Source: CAD feature listing. Evaluate the final solid. Frame: model axes, mm. Face numbers are marked on the shaded views. A direction names the side the tool comes from. Round coordinates to 2 decimals unless told otherwise and drop trailing zeros. Loops run counter-clockwise (first coordinate to the right, second up) from the corner with the lowest first, then second, coordinate; pieces in that order, holes last. Notation, with made-up numbers: (-20, -8.75) - (9, -8.75) arc R21 cw to (9, 14.25) - close; hole circle Ø6 at (83, 40.25). An arc over 180 degrees is marked (long way). One line per question, with ' | ' between items. Start each with the question number.
1. Cut plane D-D (y = -3.75). Return loops of the section in (x, z).
2. Pin query (flat end, axial travel): pin 1 (2.5 mm diameter, centred on y = -1.5, z = -14.5, fed in from -X); pin 2 (3 mm diameter, centred on x = 4.5, y = -4.5, fed in from -Z); pin 3 (13.5 mm diameter, centred on x = 42.5, z = -12, fed in from -Y); pin 4 (8 mm diameter, centred on x = 48.5, z = -15, fed in from -Y). Return the tip coordinate at first contact, or that it passes through.
3. Access query for the marked faces 1, 2 and 3. Directions: +Z, -Z, +X, -X, +Y, -Y. A direction counts if a zero-diameter tool reaches every point of the face in a straight line with its end or side. Return the directions, or none.
4. Cut plane C-C (x = 11). Return loops of the section in (y, z), then the cut area to 3 significant figures.
5. Mould query, pull axis X, two halves, no side actions, for the marked faces 4, 5 and 6. Classes: pulls with the +X half, pulls with the -X half, needs draft (parallel to the pull), parting line crosses it, or undercut.
6. Cut plane B-B (z = -25.5). Return loops of the section in (x, y), then the cut area to 3 significant figures.
7. Cut plane A-A (y = -7.5). Return loops of the section in (x, z), then the cut area to 3 significant figures.
8. Ray query, line 1 (X direction, y = -3.25, z = -22.5); line 2 (Z direction, x = 26, y = -2); line 3 (Y direction, x = 33, z = -1). Return the intervals inside material, ascending.
```python
from build123d import *

# Parameters (mm, degrees)
F1_DEPTH = 5
F2_DEPTH = 10


with BuildPart() as f1:
    # F0 (on Front) → F1 (new body)
    with BuildSketch(Plane.XZ):
        with BuildLine():
            ThreePointArc((0, -2.5), (1.767766953, -1.767766953), (2.5, 0))
            ThreePointArc((2.5, 0), (1.767766953, 1.767766953), (0, 2.5))
            Line((0, 2.5), (0, -2.5))
        make_face()
        with BuildLine():
            ThreePointArc((0, 2.5), (1.767766953, 1.767766953), (2.5, 0))
            ThreePointArc((2.5, 0), (1.767766953, -1.767766953), (0, -2.5))
            Line((0, -2.5), (28, -2.5))
            ThreePointArc((28, -2.5), (25.5, 0), (28, 2.5))
            Line((28, 2.5), (0, 2.5))
        make_face()
        with BuildLine():
            Line((0, -2.5), (0, 2.5))
            ThreePointArc((0, 2.5), (-2.5, 0), (0, -2.5))
        make_face()
        with BuildLine():
            Line((52, 2.5), (28, 2.5))
            ThreePointArc((28, 2.5), (29.767766953, 1.767766953), (30.5, 0))
            ThreePointArc((30.5, 0), (29.767766953, -1.767766953), (28, -2.5))
            Line((28, -2.5), (49.5, -2.5))
            Line((49.5, -2.5), (49.5, 0))
            ThreePointArc((49.5, 0), (50.232233047, 1.767766953), (52, 2.5))
        make_face()
        with BuildLine():
            ThreePointArc((30.5, 0), (29.767766953, 1.767766953), (28, 2.5))
            ThreePointArc((28, 2.5), (25.5, 0), (28, -2.5))
            ThreePointArc((28, -2.5), (29.767766953, -1.767766953), (30.5, 0))
        make_face()
        with BuildLine():
            Line((52, 0), (52, 2.5))
            ThreePointArc((52, 2.5), (50.232233047, 1.767766953), (49.5, 0))
            Line((49.5, 0), (52, 0))
        make_face()
        with BuildLine():
            ThreePointArc((54.5, 0), (53.767766953, 1.767766953), (52, 2.5))
            Line((52, 2.5), (52, 0))
            Line((52, 0), (54.5, 0))
        make_face()
        with BuildLine():
            Line((49.5, 0), (49.5, -2.5))
            Line((49.5, -2.5), (52, -2.5))
            ThreePointArc((52, -2.5), (50.232233047, -1.767766953), (49.5, 0))
        make_face()
        with BuildLine():
            Line((52, -2.5), (49.5, -2.5))
            Line((49.5, -2.5), (49.5, -27))
            ThreePointArc((49.5, -27), (52, -24.5), (54.5, -27))
            Line((54.5, -27), (54.5, 0))
            ThreePointArc((54.5, 0), (53.767766953, -1.767766953), (52, -2.5))
        make_face()
        with BuildLine():
            ThreePointArc((52, -2.5), (53.767766953, -1.767766953), (54.5, 0))
            Line((54.5, 0), (52, 0))
            Line((52, 0), (52, -2.5))
        make_face()
        with BuildLine():
            Line((54.5, -27), (49.5, -27))
            ThreePointArc((49.5, -27), (52, -29.5), (54.5, -27))
        make_face()
        with BuildLine():
            ThreePointArc((54.5, -27), (52, -24.5), (49.5, -27))
            Line((49.5, -27), (54.5, -27))
        make_face()
        with BuildLine():
            Line((52, 0), (49.5, 0))
            ThreePointArc((49.5, 0), (50.232233047, -1.767766953), (52, -2.5))
            Line((52, -2.5), (52, 0))
        make_face()
    extrude(amount=F1_DEPTH)

    # F0 (on Front) → F2 (join)
    with BuildSketch(Plane.XZ):
        with BuildLine():
            ThreePointArc((0, -2.5), (1.767766953, -1.767766953), (2.5, 0))
            ThreePointArc((2.5, 0), (1.767766953, 1.767766953), (0, 2.5))
            Line((0, 2.5), (0, -2.5))
        make_face()
        with BuildLine():
            Line((0, -2.5), (0, 2.5))
            ThreePointArc((0, 2.5), (-2.5, 0), (0, -2.5))
        make_face()
        with BuildLine():
            ThreePointArc((30.5, 0), (29.767766953, 1.767766953), (28, 2.5))
            ThreePointArc((28, 2.5), (25.5, 0), (28, -2.5))
            ThreePointArc((28, -2.5), (29.767766953, -1.767766953), (30.5, 0))
        make_face()
        with BuildLine():
            Line((52, 0), (49.5, 0))
            ThreePointArc((49.5, 0), (50.232233047, -1.767766953), (52, -2.5))
            Line((52, -2.5), (52, 0))
        make_face()
        with BuildLine():
            ThreePointArc((52, -2.5), (53.767766953, -1.767766953), (54.5, 0))
            Line((54.5, 0), (52, 0))
            Line((52, 0), (52, -2.5))
        make_face()
        with BuildLine():
            ThreePointArc((54.5, 0), (53.767766953, 1.767766953), (52, 2.5))
            Line((52, 2.5), (52, 0))
            Line((52, 0), (54.5, 0))
        make_face()
        with BuildLine():
            Line((52, 0), (52, 2.5))
            ThreePointArc((52, 2.5), (50.232233047, 1.767766953), (49.5, 0))
            Line((49.5, 0), (52, 0))
        make_face()
        with BuildLine():
            ThreePointArc((54.5, -27), (52, -24.5), (49.5, -27))
            Line((49.5, -27), (54.5, -27))
        make_face()
        with BuildLine():
            Line((54.5, -27), (49.5, -27))
            ThreePointArc((49.5, -27), (52, -29.5), (54.5, -27))
        make_face()
    extrude(amount=F2_DEPTH)


solid = f1.part
```
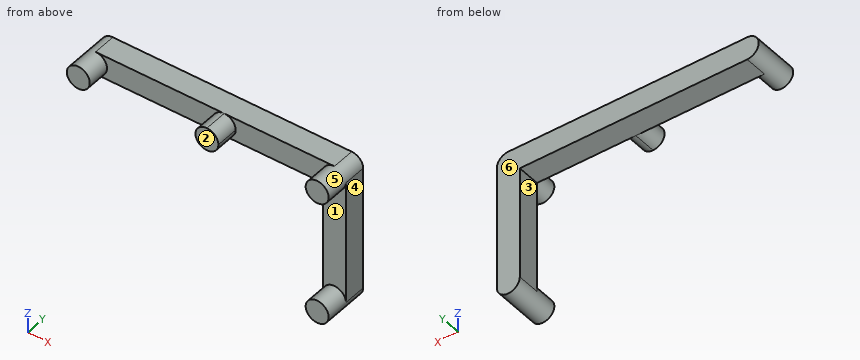
Answers follow:
1) outline: (0, -2.5) - (49.5, -2.5) - (49.5, -27) arc R2.5 ccw to (54.5, -27) - (54.5, 0) arc R2.5 ccw to (52, 2.5) - (0, 2.5) arc R2.5 ccw to start
2) pin 1: stops at x = 49.5 | pin 2: stops at z = -2.5 | pin 3: passes through | pin 4: stops at y = -5
3) face 1: -Y | face 2: +Z, -Z, +X, -X, -Y | face 3: -Z, -X, +Y, -Y
4) outline: (-5, -2.5) - (0, -2.5) - (0, 2.5) - (-5, 2.5) - close | area: 25.0 mm2
5) face 4: pulls with the +X half | face 5: undercut | face 6: needs draft
6) outline: (49.5, -5) - (50, -5) - (50, -10) - (54, -10) - (54, -5) - (54.5, -5) - (54.5, 0) - (49.5, 0) - close | area: 45.0 mm2
7) outline: circle Ø5 at (0, 0); circle Ø5 at (28, 0); circle Ø5 at (52, -27); circle Ø5 at (52, 0) | area: 78.5 mm2
8) line 1: x = 49.5 to 54.5 | line 2: z = -2.5 to 2.5 | line 3: y = -5 to 0
